Study the drawing (mm; zero at the part's minimum x, y, z) and answer. A direction names the side the tool comes from. Coordinates: 2 decimals unless noted, no trailing zeros. Order: outer loops, then holes, each group sorted by start corner. A loop starts at its lowest first (then second) coordinate and runs counter-clockwise, first axis right, second up. Notation, with made-up numbers: M -21.5,18 L 32.5,18 A29 cw 32.5,48 Z; hole C 64,50.5 d2. An arc over 180 degrees is marked long. One line per item, written item: value. Start each with the question number.
Q1. For the marked faces 1, 2 and 3, determine the directions among +Z, -Z, +X, -X, +Y, -Y from which every point of the face is accessible in a straight line to the end or side of a thin tool.
Q2. The part is cut by section C-C on y = 2.5. Give the vertices of the cut face in (x, z), then the cut area to 3 significant figures.
Q3. The part is cut by section D-D on x = 8.75. Give the vertices of the cut face in (y, z).
Q4. The part is cut by section B-B on x = 51.5. Give the vertices of the cut face in (y, z), then the cut area to 3 significant figures.
Q5. Straight lines are drawn through the part: line 1 along Z through (x, y) = (8.75, 5.45); line 2 along X through (y, z) = (0.75, 5.5); line 3 along Y through (x, z) = (7.5, 5). For each, find the intervals that lie inside material, in ascending order. Write a range as [from, to].
Q6. The part is cut by section A-A on z = 7.5. Give the vertices of the cut face in (x, y), then the cut area to 4 significant figures.
Q7. Each of these flat-tipped pins is pushed along its axis until it touches: pin 1 Ø5 at (x, z) = (8.75, 37.5) entering from -Y; pin 2 Ø2 at (y, z) = (3.5, 12) entering from -X. Where does it stop, or does it pass through?
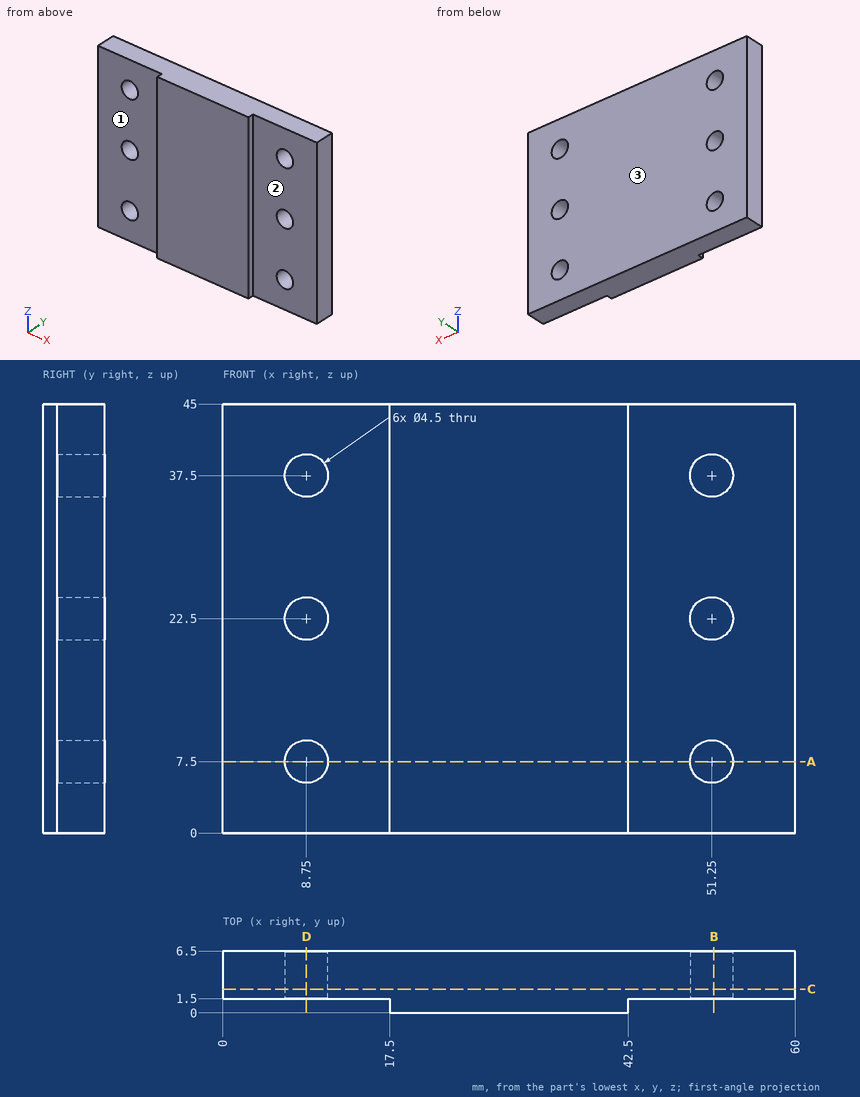
Output:
1. face 1: +Z, -Z, -X, -Y
1. face 2: +Z, -Z, +X, -Y
1. face 3: +Z, -Z, +X, -X, +Y
2. outline: M 0,0 L 60,0 L 60,45 L 0,45 Z; hole C 8.75,7.5 d4.5; hole C 8.75,22.5 d4.5; hole C 8.75,37.5 d4.5; hole C 51.25,7.5 d4.5; hole C 51.25,22.5 d4.5; hole C 51.25,37.5 d4.5
2. area: 2,600 mm^2
3. outline: M 1.5,0 L 6.5,0 L 6.5,5.25 L 1.5,5.25 Z; M 1.5,9.75 L 6.5,9.75 L 6.5,20.25 L 1.5,20.25 Z; M 1.5,24.75 L 6.5,24.75 L 6.5,35.25 L 1.5,35.25 Z; M 1.5,39.75 L 6.5,39.75 L 6.5,45 L 1.5,45 Z
4. outline: M 1.5,0 L 6.5,0 L 6.5,5.26 L 1.5,5.26 Z; M 1.5,9.74 L 6.5,9.74 L 6.5,20.26 L 1.5,20.26 Z; M 1.5,24.74 L 6.5,24.74 L 6.5,35.26 L 1.5,35.26 Z; M 1.5,39.74 L 6.5,39.74 L 6.5,45 L 1.5,45 Z
4. area: 158 mm^2
5. line 1: z = [0, 5.25], [9.75, 20.25], [24.75, 35.25], [39.75, 45]
5. line 2: x = [17.5, 42.5]
5. line 3: y = [1.5, 6.5]
6. outline: M 0,1.5 L 6.5,1.5 L 6.5,6.5 L 0,6.5 Z; M 11,1.5 L 17.5,1.5 L 17.5,0 L 42.5,0 L 42.5,1.5 L 49,1.5 L 49,6.5 L 11,6.5 Z; M 53.5,1.5 L 60,1.5 L 60,6.5 L 53.5,6.5 Z
6. area: 292.5 mm^2
7. pin 1: stops at y = 1.5
7. pin 2: stops at x = 0
